Geometry: final body of the model. Coordinates: model frame, mm. Give positions to 0.01 mm unless a question says otherwise; leave off trailing zeros. Write each loop counter-clockwise with the first axis right and the second up, starting at its lowest first coordinate (ties: lowest second). Pieces come first, ordered by that corner, then holes. Notation, with made-up numbers: M -39.5,25 L -3.5,25 A23 cw -3.5,45 Z; hole C 70,66 d2. An arc over 180 degrees is marked long. Use a Markdown table: item, result. Add a question column.
(1) Material intervals for L1, parallel to Z at x = 1327.5, y = 23.75; L2, parallel to Y at x = 712.5, z = -16; L3, parallel to Z at x = 324, y = 2.75, sorted ascending.
(2) Pin query (flat end, axial travel): pin 1 Ø6.5 at (x, z) = (12.7, -22.225) entering from +Y; pin 2 Ø4 at (x, z) = (1241.425, -22.225) entering from -Y; pin 3 Ø1.5 at (x, y) = (460, 3) entering from -Z; pin 4 Ø6 at (x, z) = (1522, -39) entering from +Y. Return the tip coordinate at first contact, or that it passes through.
(3) Cut plane A-A (x = 576.5). Output: boundary loops of the cut face in (y, z) (3 decimals).
(4) Cut plane B-B (z = -12.5). Output: boundary loops of the cut face in (x, y), plus the area to 3 significant figures.
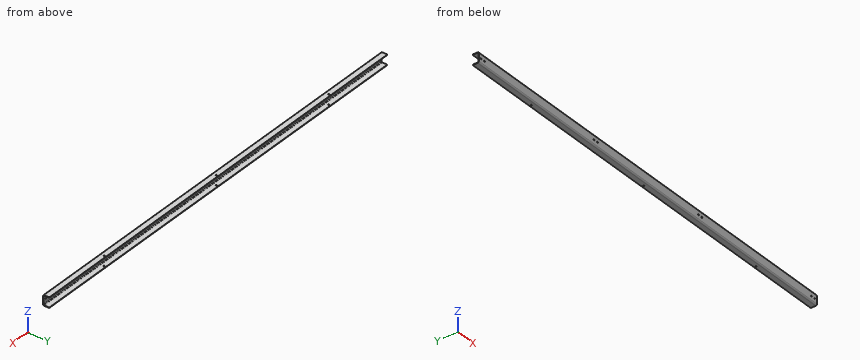
```python
from build123d import *

# Parameters (mm, degrees)
BASE_FLANGE1_DEPTH = 1911.35
SKETCH2_R          = 2.4511
CUT_EXTRUDE1_DEPTH = 1913.06358148
SKETCH3_R          = 2.4511
CUT_EXTRUDE2_DEPTH = 1913.06358148
FILLET1_R          = 3.175


# Sheet-metal steps are written as plain solids
with BuildPart() as part:
    # Sketch1 → Base-Flange1 (new body)
    with BuildSketch(Plane(origin=(0, 0, 0), x_dir=(0, 0, -1), z_dir=(1, 0, 0))):
        with BuildLine():
            Line((0, 27.432), (0, 5.207))
            ThreePointArc((0, 5.207), (1.52509499, 1.52509499), (5.207, 0))
            Line((5.207, 0), (39.243, 0))
            ThreePointArc((39.243, 0), (42.92490501, 1.52509499), (44.45, 5.207))
            Line((44.45, 5.207), (44.45, 27.432))
            Line((44.45, 27.432), (42.418, 27.432))
            Line((42.418, 27.432), (42.418, 5.207))
            ThreePointArc((42.418, 5.207), (41.48806403, 2.96193597), (39.243, 2.032))
            Line((39.243, 2.032), (5.207, 2.032))
            ThreePointArc((5.207, 2.032), (2.96193597, 2.96193597), (2.032, 5.207))
            Line((2.032, 5.207), (2.032, 27.432))
            Line((2.032, 27.432), (0, 27.432))
        make_face()
    extrude(amount=BASE_FLANGE1_DEPTH)

    # Sketch2 → Cut-Extrude1 (cut, through all)
    with BuildSketch(Plane(origin=(0, 0, 0), x_dir=(-1, 0, 0), z_dir=(0, -1, 0))):
        with Locations(Location((-12.7, 22.225, 0), (0, 0, 90))):
            Circle(SKETCH2_R)
        with Locations(Location((-31.75, 22.225, 0), (0, 0, 90))):
            Circle(SKETCH2_R)
        with Locations(Location((-650.875, 22.225, 0), (0, 0, 90))):
            Circle(SKETCH2_R)
        with Locations(Location((-669.925, 22.225, 0), (0, 0, 90))):
            Circle(SKETCH2_R)
        with Locations(Location((-1898.65, 22.225, 0), (0, 0, 270))):
            Circle(SKETCH2_R)
        with Locations(Location((-1879.6, 22.225, 0), (0, 0, 270))):
            Circle(SKETCH2_R)
        with Locations(Location((-1260.475, 22.225, 0), (0, 0, 270))):
            Circle(SKETCH2_R)
        with Locations(Location((-1241.425, 22.225, 0), (0, 0, 270))):
            Circle(SKETCH2_R)
    extrude(amount=-CUT_EXTRUDE1_DEPTH, mode=Mode.SUBTRACT)

    # Sketch3 → Cut-Extrude2 (cut, through all)
    with BuildSketch(Plane(origin=(0, 0, -44.45), x_dir=(-1, 0, 0), z_dir=(0, 0, -1))):
        with Locations((-1590.675, 19.05)):
            Circle(SKETCH3_R)
        with Locations((-955.675, 19.05)):
            Circle(SKETCH3_R)
        with Locations((-320.675, 19.05)):
            Circle(SKETCH3_R)
    extrude(amount=-CUT_EXTRUDE2_DEPTH, mode=Mode.SUBTRACT)

    # Fillet1
    fillet1_edges = [part.edges().sort_by_distance(p)[0] for p in [
        (0, 27.432, -1.016),
        (0, 27.432, -43.434),
        (1911.35, 27.432, -1.016),
        (1911.35, 27.432, -43.434),
    ]]
    fillet(fillet1_edges, radius=FILLET1_R)


solid = part.part
```
Answer list:
| question | item | result |
|---|---|---|
| 1 | L1 | -44.45 to -42.42, -2.03 to 0 |
| 1 | L2 | 0 to 2.03 |
| 1 | L3 | -43.83 to -41.25, -3.2 to -0.62 |
| 2 | pin 1 | y = 2.03 |
| 2 | pin 2 | through |
| 2 | pin 3 | z = -44.24 |
| 2 | pin 4 | y = 3.63 |
| 3 | outline | M 0,-39.243 A5.207 ccw 5.207,-44.45 L 27.432,-44.45 L 27.432,-42.418 L 5.207,-42.418 A3.175 cw 2.032,-39.243 L 2.032,-5.207 A3.175 cw 5.207,-2.032 L 27.432,-2.032 L 27.432,0 L 5.207,0 A5.207 ccw 0,-5.207 Z |
| 4 | outline | M 0,0 L 1911.35,0 L 1911.35,2.03 L 0,2.03 Z |
| 4 | area | 3,880 mm² |
